Autodesk Inventor part; units mm, degrees
ref_plane "FOR_P2_XY" through (0, 56.2, 0) normal (0, 1, 0) x (1, 0, 0)
ref_plane "FOR_P2_YZ" through (0, 56.2, 0) normal (1, 0, 0) x (0, 0, -1)
ref_plane "FOR_P2_ZX" through (0, 56.2, 0) normal (0, 0, -1) x (0, 1, 0)
sketch "Sketch_1" plane through (0, 0, 0) normal (1, 0, 0) x (0, 1, 0)
  line L0 (-30.3, 73) -> (-30.3, 68)
  line L1 (-30.3, 68) -> (-56.2, 68)
  line L2 (-56.2, 68) -> (-56.2, 0)
  line L3 (-56.2, 0) -> (56.2, 0)
  line L4 (56.2, 0) -> (56.2, 68)
  line L5 (56.2, 68) -> (14.7, 68)
  line L6 (14.7, 68) -> (14.7, 73)
  line L7 (14.7, 73) -> (-30.3, 73)
extrude "Extrusion1" add sketch "Sketch_1" along normal blind 90
sketch "Sketch_3" plane through (45, 0, 0) normal (1, 0, 0) x (0, 0, -1)
  line L0 (-69, -56.2) -> (-65.75, -56.2)
  line L1 (-65.75, -56.2) -> (-66, -55.95)
  line L2 (-66, -55.95) -> (-66, -36.15)
  line L3 (-66, -36.15) -> (-69, -36.15)
  line L4 (-69, -36.15) -> (-69, -56.2)
extrude "Extrusion2" cut sketch "Sketch_3" along normal mid plane 79.1
sketch "Sketch_2" plane through (45, 0, 0) normal (1, 0, 0) x (0, 0, -1)
  line L0 (-68.007, -56.2) -> (-66, -56.2)
  line L1 (-66, -56.2) -> (-66, -36.4)
  line L2 (-66, -36.4) -> (-68.007, -36.4)
  line L3 (-68.007, -36.4) -> (-68.007, -56.2)
extrude "Extrusion3" add sketch "Sketch_2" along normal mid plane 78.6
sketch "Sketch_4" plane through (35.991, 0, 0) normal (1, 0, 0) x (0, 0, -1)
  arc A0 (-73, 11.7765) -> (-73, -27.3765) centre (-0.6, -7.8) ccw
  line L0 (-73, -27.3765) -> (-73, 11.7765)
extrude "Extrusion4" add sketch "Sketch_4" against normal blind 2.182
sketch "Sketch_5" plane through (54.009, 0, 0) normal (1, 0, 0) x (0, 0, -1)
  arc A0 (-73, 11.7765) -> (-73, -27.3765) centre (-0.6, -7.8) ccw
  line L0 (-73, -27.3765) -> (-73, 11.7765)
extrude "Extrusion5" add sketch "Sketch_5" along normal blind 2.182
sketch "Sketch_7" plane through (0, 0, 21) normal (0, 0, 1) x (1, 0, 0)
  line L0 (8.9, -71.05) -> (21.1, -71.05)
  line L1 (21.1, -71.05) -> (21.1, -54.2)
  line L2 (21.1, -54.2) -> (38.9, -54.2)
  line L3 (38.9, -54.2) -> (38.9, -71.05)
  line L4 (38.9, -71.05) -> (51.1, -71.05)
  line L5 (51.1, -71.05) -> (51.1, -54.2)
  line L6 (51.1, -54.2) -> (68.9, -54.2)
  line L7 (68.9, -54.2) -> (68.9, -71.05)
  line L8 (68.9, -71.05) -> (81.1, -71.05)
  line L9 (81.1, -71.05) -> (81.1, 71.05)
  line L10 (81.1, 71.05) -> (68.9, 71.05)
  line L11 (68.9, 71.05) -> (68.9, 54.2)
  line L12 (68.9, 54.2) -> (51.1, 54.2)
  line L13 (51.1, 54.2) -> (51.1, 71.05)
  line L14 (51.1, 71.05) -> (38.9, 71.05)
  line L15 (38.9, 71.05) -> (38.9, 54.2)
  line L16 (38.9, 54.2) -> (21.1, 54.2)
  line L17 (21.1, 54.2) -> (21.1, 71.05)
  line L18 (21.1, 71.05) -> (8.9, 71.05)
  line L19 (8.9, 71.05) -> (8.9, -71.05)
  circle A0 centre (75, 64.05) radius 3.25
  circle A1 centre (75, -64.05) radius 3.25
  circle A2 centre (45, 64.05) radius 3.25
  circle A3 centre (45, -64.05) radius 3.25
  circle A4 centre (15, 64.05) radius 3.25
  circle A5 centre (15, -64.05) radius 3.25
extrude "Extrusion6" add sketch "Sketch_7" against normal blind 2
ref_plane "FOR_P2_XY" through (0, 56.2, 0) normal (0, 1, 0) x (1, 0, 0)
ref_plane "FOR_P2_YZ" through (0, 56.2, 0) normal (1, 0, 0) x (0, 0, -1)
ref_plane "FOR_P2_ZX" through (0, 56.2, 0) normal (0, 0, -1) x (0, 1, 0)
ref_plane "FOR_P22_XY" through (90, -56.2, 0) normal (0, -1, 0) x (1, 0, 0)
ref_plane "FOR_P22_YZ" through (90, -56.2, 0) normal (1, 0, 0) x (0, 0, 1)
ref_plane "FOR_P22_ZX" through (90, -56.2, 0) normal (0, 0, 1) x (0, -1, 0)
ref_plane "P1_XY" through (0, 0, 0) normal (0, 0, 1) x (1, 0, 0)
ref_plane "P1_YZ" through (0, 0, 0) normal (1, 0, 0) x (0, 1, 0)
ref_plane "P1_ZX" through (0, 0, 0) normal (0, 1, 0) x (0, 0, 1)
ref_plane "P3_XY" through (45, -5.518, 73) normal (0, 0, 1) x (1, 0, 0)
ref_plane "P3_YZ" through (45, -5.518, 73) normal (1, 0, 0) x (0, 1, 0)
ref_plane "P3_ZX" through (45, -5.518, 73) normal (0, 1, 0) x (0, 0, 1)
properties part number "nzm1_3p_p1"
For this review, take the finished solid that the model builds, in its own axes (mm). A direction names the side the tool comes from. Give positions to 0.01 mm unless a question says otherwise; leave off trailing zeros. Write each loop counter-clockwise with the first axis right and the second up, starting at its lowest first coordinate (ties: lowest second). Pieces come first, ordered by that corner, then holes. Notation, with made-up numbers: M -28,75.25 L -20,75.25 A22 ccw -20,107.25 Z; hole C 69.5,76.25 d10. An arc over 180 degrees is marked long. Answer as a JSON object with one key per item and string values. Group by question number.
Item 1: Consider section D-D on y = -40.5. Write out the cut boundary in (x, z).
Item 2: For pin 1 Ø1 at (y, z) = (66, 20) entering from +X; pin 2 Ø3 at (x, z) = (75.5, 57.5) entering from -Y; pin 3 Ø1 at (y, z) = (60.5, 20) entering from -X, all flat-tipped, find the tip position at first contact; note any pin that passes through.
Item 3: Tool access review of faces 5 (the flat face through (18, -62, 21)), 6 (the flat face through (42, -62, 19)), 7 (the flat face through (12, 62, 19)): name each direction out of +Z, -Z, +X, -X, +Y, -Y from which nothing blocks a thin tool from reaching the whole face with its end or side.
Item 4: Consider section A-A on x = 75. Count the separate pieces of the cut face and the enclosed holes in it, plus the area to 3 significant figures.
Item 5: Draft analysis for pull direction X (two halves, no side actions). For faces 1 (the flat face through (0, -1, 37)), 2 (the flat face through (44, -1, 0)), 3 (the cylindrical face through (48.1, -63.07, 20.01)), 4 (the cylindrical face through (14.295, 60.877, 20.014)), state which applies: +X half, -X half, draft (parallel to the pull), parting line (faces both ways), or undercut.
Item 6: Consider section C-C on x = 62. Write out the cut boundary in (y, z), plus the area to 3 significant figures.
Item 7: Consider section B-B on y = -64.05. Write out the cut boundary in (x, z), plus the area to 3 significant figures.
Item 8: For probe 1 along Y at (x, z) = (45, 20); probe 2 along Z at (x, y) = (79, 43.5); probe 3 along Y at (x, z) = (69, 56), list the stretches that pass through material, from the lowest coordinate up. Write a range as [from, to].
Check result:
{
 "1": {"outline": "M 0,0 L 90,0 L 90,68 L 84.55,68 L 84.55,66 L 84.3,66 L 84.3,68.01 L 5.7,68.01 L 5.7,66 L 5.45,66 L 5.45,68 L 0,68 Z"},
 "2": {"pin 1": "stops at x = 81.1", "pin 2": "stops at y = -56.2", "pin 3": "stops at x = 8.9"},
 "3": {"face 5": "+Z, +X, -X, -Y", "face 6": "-Z, +X, -X, -Y", "face 7": "-Z, +X, -X, +Y"},
 "4": {"separate pieces": "3", "enclosed holes": "0", "area": "7,900 mm^2"},
 "5": {"face 1": "-X half", "face 2": "draft", "face 3": "undercut", "face 4": "undercut"},
 "6": {"outline": "M -56.2,0 L 56.2,0 L 56.2,68 L 14.7,68 L 14.7,73 L -30.3,73 L -30.3,68 L -36.15,68 L -36.15,66 L -36.4,66 L -36.4,68.01 L -56.2,68.01 L -56.2,66 L -55.95,66 L -56.2,65.75 Z", "area": "7,870 mm^2"},
 "7": {"outline": "M 8.9,19 L 11.75,19 L 11.75,21 L 8.9,21 Z; M 18.25,19 L 21.1,19 L 21.1,21 L 18.25,21 Z; M 38.9,19 L 41.75,19 L 41.75,21 L 38.9,21 Z; M 48.25,19 L 51.1,19 L 51.1,21 L 48.25,21 Z; M 68.9,19 L 71.75,19 L 71.75,21 L 68.9,21 Z; M 78.25,19 L 81.1,19 L 81.1,21 L 78.25,21 Z", "area": "34.2 mm^2"},
 "8": {"probe 1": "y = [-71.05, -67.3], [-60.8, 60.8], [67.3, 71.05]", "probe 2": "z = [0, 68]", "probe 3": "y = [-56.2, 56.2]"}
}
